Input: dimensioned drawing with shaded views. Units: mm. Origin: part minimum x, y, z. Coordinates: 2 decimals unless noted, no trailing zeros. Write each loop counter-clockwise with the first axis right and the second up, starting at its lowest first coordinate (ties: lowest second). Pieces come first, ordered by that corner, then holes. Notation, with made-up numbers: (27, 52) - (33, 52) arc R31 ccw to (33, 90) - close; hole circle Ø10 at (6.25, 4). An arc over 180 degrees is marked (long way). One line per question, with ' | ' between items.
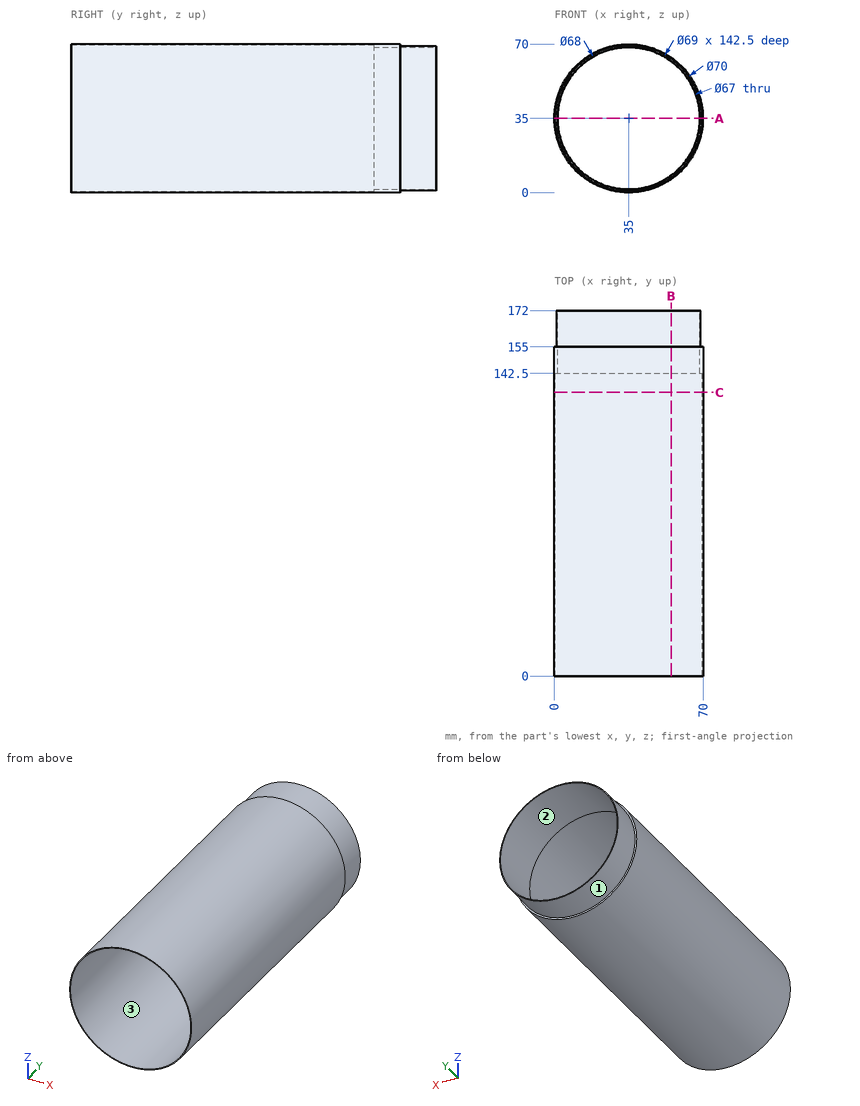
Item 1: Mould query, pull axis X, two halves, no side actions, for the marked faces 1, 2 and 3. Classes: pulls with the +X half, pulls with the -X half, needs draft (parallel to the pull), parting line crosses it, or undercut.
Check sheet entries:
face 1: parting line crosses it | face 2: undercut | face 3: undercut
Item 2: Cut plane A-A on z = 35. Return loops of the section in (x, y).
Check sheet entries:
outline: (0, 0) - (0.5, 0) - (0.5, 142.5) - (1.5, 142.5) - (1.5, 172) - (1, 172) - (1, 155) - (0, 155) - close; (68.5, 142.5) - (69.5, 142.5) - (69.5, 0) - (70, 0) - (70, 155) - (69, 155) - (69, 172) - (68.5, 172) - close
Item 3: Ray query, line 1 along Z through (x, y) = (35, 152); line 2 along Z through (x, y) = (35, 164); line 3 along X through (y, z) = (150, 43). Return the intervals inside material, ascending. Write a range as [from, to].
Check sheet entries:
line 1: [0, 1.5], [68.5, 70] | line 2: [1, 1.5], [68.5, 69] | line 3: [0.93, 2.47], [67.53, 69.07]
Item 4: Pin query (flat end, axial travel): pin 1 Ø8 at (y, z) = (105.5, 14) entering from -X; pin 2 Ø6 at (x, y) = (8, 85) entering from -Z; pin 3 Ø3 at (y, z) = (148, 32) entering from +X. Return the tip coordinate at first contact, or that it passes through.
Check sheet entries:
pin 1: x = 4.41 | pin 2: z = 9.52 | pin 3: x = 69.97
Item 5: Cut plane C-C on y = 133.5. Return loops of the section in (x, z), and give its area (3 significant figures).
Check sheet entries:
outline: circle Ø70 at (35, 35); hole circle Ø69 at (35, 35) | area: 109 mm²
Item 6: Cut plane B-B on x = 55. Return loops of the section in (y, z).
Check sheet entries:
outline: (0, 6.28) - (155, 6.28) - (155, 7.5) - (172, 7.5) - (172, 8.13) - (142.5, 8.13) - (142.5, 6.89) - (0, 6.89) - close; (0, 63.11) - (142.5, 63.11) - (142.5, 61.87) - (172, 61.87) - (172, 62.5) - (155, 62.5) - (155, 63.72) - (0, 63.72) - close
